Geometry: final body of the model. Coordinates: model frame, mm. Round coordinates to 2 decimals unless told otherwise and drop trailing zeros. Loops run counter-clockwise (first coordinate to the right, second up) from the corner with the lowest first, then second, coordinate; pieces in that order, holes last. Notation, with made-up numbers: M 84,32 L 136,32 A15 cw 136,47 Z; hole C 61.5,68 d10. An arc over 180 degrees is marked long. Answer as a JSON object with one key per item and string values.
Autodesk Fusion 360 part; units mm, degrees
sketch "Sketch1" plane through (0, 0, 0) normal (0, 0, 1) x (1, 0, 0)
  line L0 (-45, 50) -> (25, 50)
  line L1 (25, 50) -> (25, -50)
  line L2 (25, -50) -> (-45, -50)
  line L3 (-45, -50) -> (-45, 50)
  dimension "d1" = 70
  dimension "d2" = 100
extrude "Extrude1" add sketch "Sketch1" along normal blind 40
sketch "Sketch2" plane through (0, 0, 40) normal (0, 0, 1) x (-1, 0, 0)
  line L0 (45, 50) -> (-25, 50)
  line L1 (-25, 50) -> (-25, -50)
  line L2 (-25, -50) -> (45, -50)
  line L3 (45, -50) -> (45, 50)
  line L4 (40, -50) -> (40, 50) construction
  line L5 (30, -50) -> (30, 50) construction
  line L6 (20, -50) -> (20, 50) construction
  line L7 (10, -50) -> (10, 50) construction
  line L8 (0, -50) -> (0, 50) construction
  line L9 (-15, -50) -> (-15, 50) construction
  line L10 (45, -40) -> (-25, -40) construction
  line L11 (45, -30) -> (-25, -30) construction
  line L12 (45, -20) -> (-25, -20) construction
  line L13 (45, -10) -> (-25, -10) construction
  line L14 (45, 35) -> (-25, 35) construction
  line L15 (45, 45) -> (-25, 45) construction
  circle A0 centre (40, -40) radius 1.5
  circle A1 centre (40, -30) radius 1.5
  circle A2 centre (40, -20) radius 1.5
  circle A3 centre (40, -10) radius 1.5
  line L16 (45, 0) -> (-25, 0) construction
  line L17 (45, 10) -> (-25, 10) construction
  line L18 (45, 20) -> (-25, 20) construction
  line L19 (45, 30) -> (-25, 30) construction
  line L20 (-25, 42) -> (45, 42) construction
  circle A4 centre (40, 0) radius 1.5 construction
  circle A5 centre (40, 0) radius 1.5
  circle A6 centre (40, 10) radius 1.5
  circle A7 centre (40, 20) radius 1.5
  circle A8 centre (30, 0) radius 1.5
  circle A9 centre (30, -30) radius 1.5
  circle A10 centre (30, 20) radius 1.5
  circle A11 centre (30, 0) radius 1.5 construction
  circle A12 centre (30, -40) radius 1.5
  circle A13 centre (30, -20) radius 1.5
  circle A14 centre (30, 10) radius 1.5
  circle A15 centre (30, -10) radius 1.5
  circle A16 centre (0, -40) radius 2.5
  circle A17 centre (0, -30) radius 2.5
  circle A18 centre (0, -20) radius 2.5
  circle A19 centre (0, -10) radius 2.5
  circle A20 centre (0, 10) radius 2.5
  circle A21 centre (0, 0) radius 2.5
  circle A22 centre (0, 10) radius 2.5
  circle A23 centre (0, 20) radius 2.5
  circle A24 centre (10, 0) radius 2.5
  circle A25 centre (10, 10) radius 2.5
  circle A26 centre (10, 20) radius 2.5
  circle A27 centre (10, 10) radius 2.5
  circle A28 centre (10, -40) radius 2.5
  circle A29 centre (10, -20) radius 2.5
  circle A30 centre (10, -10) radius 2.5
  circle A31 centre (10, -30) radius 2.5
  circle A32 centre (20, 0) radius 2.5
  circle A33 centre (20, 10) radius 2.5
  circle A34 centre (20, 20) radius 2.5
  circle A35 centre (20, 10) radius 2.5
  circle A36 centre (20, -40) radius 2.5
  circle A37 centre (20, -20) radius 2.5
  circle A38 centre (20, -10) radius 2.5
  circle A39 centre (20, -30) radius 2.5
  circle A40 centre (-15, -40) radius 3.5
  circle A41 centre (-15, -30) radius 3.5
  circle A42 centre (-15, -20) radius 3.5
  circle A43 centre (-15, 0) radius 3.5
  circle A44 centre (-15, -10) radius 3.5
  circle A45 centre (-15, 10) radius 3.5
  circle A46 centre (-15, 20) radius 3.5
  circle A47 centre (35.1971, 30) radius 4.5
  circle A48 centre (10.1971, 30) radius 4.5
  circle A49 centre (-14.8029, 30) radius 4.5
  circle A50 centre (35, 42) radius 6
  circle A51 centre (0, 42) radius 6
  circle A52 centre (20, 42) radius 6
  circle A53 centre (-15, 42) radius 6
  circle A54 centre (35.1971, 30) radius 4.5
  circle A55 centre (22.6971, 30) radius 4.5
  circle A56 centre (-2.3029, 30) radius 4.5
  point P0 (10, -50)
  point P1 (10, 0)
  point P2 (20, -50)
  point P3 (20, 0)
  point P4 (-15, -20)
  dimension "d5" = 3
  dimension "d6" = 3
  dimension "d7" = 3
  dimension "d8" = 3
  dimension "d9" = 3
  dimension "d10" = 3
  dimension "d11" = 3
  dimension "d12" = 3
  dimension "d13" = 3
  dimension "d14" = 3
  dimension "d15" = 3
  dimension "d16" = 3
  dimension "d17" = 3
  dimension "d18" = 3
  dimension "d19" = 3
  dimension "d20" = 3
  dimension "d39" = 5
  dimension "d40" = 5
  dimension "d41" = 5
  dimension "d42" = 5
  dimension "d43" = 5
  dimension "d44" = 5
  dimension "d45" = 5
  dimension "d46" = 5
  dimension "d47" = 5
  dimension "d48" = 5
  dimension "d49" = 5
  dimension "d50" = 5
  dimension "d51" = 5
  dimension "d52" = 5
  dimension "d53" = 5
  dimension "d54" = 5
  dimension "d55" = 5
  dimension "d56" = 5
  dimension "d57" = 5
  dimension "d58" = 5
  dimension "d59" = 5
  dimension "d60" = 5
  dimension "d61" = 5
  dimension "d62" = 5
  dimension "d63" = 7
  dimension "d64" = 7
  dimension "d65" = 7
  dimension "d66" = 7
  dimension "d67" = 7
  dimension "d68" = 7
  dimension "d69" = 7
  dimension "d70" = 9
  dimension "d71" = 9
  dimension "d72" = 9
  dimension "d73" = 12
  dimension "d74" = 12
  dimension "d75" = 12
  dimension "d76" = 12
  dimension "d77" = 9
  dimension "d78" = 9
  dimension "d79" = 9
extrude "Extrude2" add sketch "Sketch2" along normal blind 20
sketch "Sketch3" plane through (0, 0, 60) normal (0, 0, 1) x (-1, 0, 0)
  circle A0 centre (-2.3029, 30) radius 4.5
  circle A1 centre (35.1971, 30) radius 4.5
  circle A2 centre (22.6971, 30) radius 4.5
  circle A3 centre (20, 42) radius 6
  circle A4 centre (0, 42) radius 6
  circle A5 centre (-15, 42) radius 6
  circle A6 centre (-15, 10) radius 3.5
  circle A7 centre (-14.8029, 30) radius 4.5
  circle A8 centre (35, 42) radius 6
  circle A9 centre (10, -40) radius 2.5
  circle A10 centre (30, -20) radius 1.5
  circle A11 centre (30, 10) radius 1.5
  circle A12 centre (30, -10) radius 1.5
  circle A13 centre (0, -40) radius 2.5
  circle A14 centre (0, -30) radius 2.5
  circle A15 centre (0, -20) radius 2.5
  circle A16 centre (0, -10) radius 2.5
  circle A17 centre (0, 0) radius 2.5
  circle A18 centre (0, 20) radius 2.5
  circle A19 centre (10, -30) radius 2.5
  circle A20 centre (20, 0) radius 2.5
  circle A21 centre (10, 20) radius 2.5
  circle A22 centre (10, 0) radius 2.5
  circle A23 centre (0, 10) radius 2.5
  circle A24 centre (10, -20) radius 2.5
  circle A25 centre (10, -10) radius 2.5
  circle A26 centre (-15, -10) radius 3.5
  circle A27 centre (30, -40) radius 1.5
  circle A28 centre (20, 20) radius 2.5
  circle A29 centre (40, 20) radius 1.5
  circle A30 centre (20, 10) radius 2.5
  circle A31 centre (30, 20) radius 1.5
  circle A32 centre (-15, -20) radius 3.5
  circle A33 centre (40, -20) radius 1.5
  circle A34 centre (40, -40) radius 1.5
  circle A35 centre (30, -30) radius 1.5
  circle A36 centre (-15, 0) radius 3.5
  circle A37 centre (10, 10) radius 2.5
  circle A38 centre (30, 0) radius 1.5
  circle A39 centre (20, -30) radius 2.5
  circle A40 centre (-15, -30) radius 3.5
  circle A41 centre (40, 10) radius 1.5
  circle A42 centre (40, -10) radius 1.5
  circle A43 centre (40, 0) radius 1.5
  circle A44 centre (20, -40) radius 2.5
  circle A45 centre (20, -20) radius 2.5
  circle A46 centre (40, -30) radius 1.5
  circle A47 centre (-15, -40) radius 3.5
  circle A48 centre (20, -10) radius 2.5
  circle A49 centre (-15, 20) radius 3.5
  circle A50 centre (10.1971, 30) radius 4.5
  line L0 (45, -50) -> (45, 50)
  line L1 (45, 50) -> (-25, 50)
  line L2 (-25, 50) -> (-25, -50)
  line L3 (-25, -50) -> (45, -50)
extrude "Extrude3" cut 1 faces at (-21.6667, 16.6667, 0) along direction (0, 0, 1) blind 15
sketch "Sketch4" plane through (0, 0, 15) normal (0, 0, -1) x (1, 0, 0)
  line L0 (25, 50) -> (-45, 50)
  line L1 (-45, 50) -> (-45, -50)
  line L2 (-45, -50) -> (25, -50)
  line L3 (25, -50) -> (25, 50)
  line L4 (-25, -50) -> (-45, -50)
  line L5 (-45, -50) -> (-45, 15)
  line L6 (-45, 15) -> (-25, 15)
  line L7 (-25, 15) -> (-25, -50)
extrude "Extrude4" add sketch "Sketch4" against normal blind 35 contours L1 L2 L4 L5 L6 L7
sketch "Sketch5" plane through (0, 0, 15) normal (0, 0, -1) x (1, 0, 0)
  line L0 (-45, -50) -> (25, -50)
  line L1 (25, -50) -> (25, 50)
  line L2 (25, 50) -> (-45, 50)
  line L3 (-45, 50) -> (-45, -50)
  line L4 (-25, -50) -> (-25, -70)
  line L5 (-25, -70) -> (-15, -75)
  line L6 (5, -50) -> (5, -65)
  line L7 (-45, 23.0126) -> (-75, 23.0126)
  line L8 (5, -50) -> (-25, -50)
  line L9 (-25, -50) -> (-25, 23.0126)
  line L10 (-25, 23.0126) -> (5, 23.0126)
  line L11 (5, 23.0126) -> (5, -50)
  dimension "d86" = 11.1803
extrude "Extrude5" add sketch "Sketch5" against normal blind 25 contours L0 L8 L9 L10 L11
extrude "Extrude6" cut 1 faces at (1.6667, 16.6667, 15) along direction (0, 0, 1) blind 20
1) Pull-direction query (Y, two-part tool) for faces 1 (the flat face through (-17, -1, 60)), 2 (the cylindrical face through (-38.5, 0.07, 54.93)); classes: +Y half, -Y half, draft (parallel to the pull), parting line (faces both ways), or undercut.
Results:
{"face 1": "draft", "face 2": "undercut"}
2) Section query B-B (z = 43.75). Count the separate pieces of the cut face and the enclosed holes in it, and give its area (3 significant figures).
Results:
{"separate pieces": "1", "enclosed holes": "39", "area": "5,530 mm2"}
3) Section query D-D (y = -30). Return the cut outline in (x, z), and give its area (3 significant figures).
Results:
{"outline": "M -45,35 L 25,35 L 25,60 L 19.3,60 L 19.3,40 L 10.3,40 L 10.3,60 L 6.8,60 L 6.8,40 L -2.2,40 L -2.2,60 L -5.7,60 L -5.7,40 L -14.7,40 L -14.7,60 L -18.2,60 L -18.2,40 L -27.2,40 L -27.2,60 L -30.7,60 L -30.7,40 L -39.7,40 L -39.7,60 L -45,60 Z", "area": "850 mm2"}
4) Section query A-A (y = 30). Return the cut outline in (x, z).
Results:
{"outline": "M -45,35 L 25,35 L 25,60 L 18.5,60 L 18.5,40 L 11.5,40 L 11.5,60 L 2.5,60 L 2.5,40 L -2.5,40 L -2.5,60 L -7.5,60 L -7.5,40 L -12.5,40 L -12.5,60 L -17.5,60 L -17.5,40 L -22.5,40 L -22.5,60 L -28.5,60 L -28.5,50 L -31.5,50 L -31.5,60 L -38.5,60 L -38.5,50 L -41.5,50 L -41.5,60 L -45,60 Z"}
5) Ray query, line 1 (X direction, y = -30, z = 51.5); line 2 (Y direction, x = -23.5, z = 41.5); line 3 (Y direction, x = -32.5, z = 51). Return the intervals inside material, ascending.
Results:
{"line 1": "-45 to -39.7, -30.7 to -27.2, -18.2 to -14.7, -5.7 to -2.2, 6.8 to 10.3, 19.3 to 25", "line 2": "-50 to -46.87, -37.13 to -34.43, -25.57 to 50", "line 3": "-50 to -47.45, -36.55 to -33.6, -26.4 to 50"}
6) Section query C-C (x = -35). Return the cut outline in (y, z).
Results:
{"outline": "M -50,35 L 50,35 L 50,60 L -25.5,60 L -25.5,40 L -34.5,40 L -34.5,60 L -36,60 L -36,40 L -48,40 L -48,60 L -50,60 Z"}
7) Pin query (flat end, axial travel): P1, Ø4, axis at x = -10, y = -10, coming from the +Z side; P2, Ø1.5, axis at x = -30.5, y = 19.5, coming from the +Z side. Return the tip coordinate at first contact, or that it passes through.
Results:
{"P1": "z = 40", "P2": "z = 50"}
